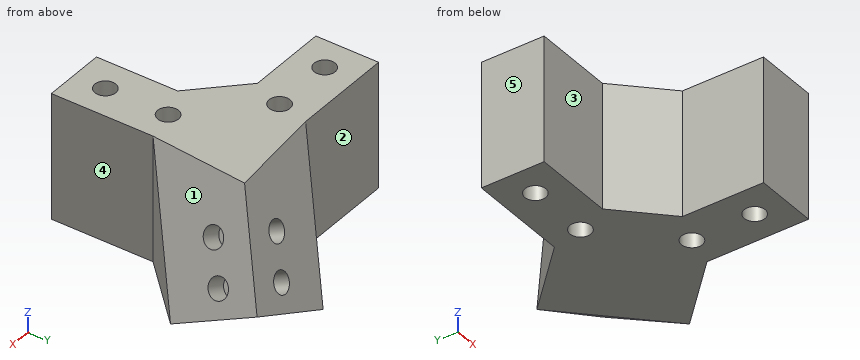
Autodesk Inventor part; units mm, degrees
ref_plane "YZ Plane" through (0, 0, 0) normal (1, 0, 0) x (0, 1, 0)
ref_plane "XZ Plane" through (0, 0, 0) normal (0, 1, 0) x (-1, 0, 0)
ref_plane "XY Plane" through (0, 0, 0) normal (0, 0, 1) x (1, 0, 0)
sketch "スケッチ1" plane through (0, 0, 0) normal (0, 0, 1) x (1, 0, 0)
  line L0 (0, 0) -> (60, 0)
  line L1 (60, 0) -> (60, 60)
  line L2 (60, 60) -> (0, 60)
  line L3 (0, 60) -> (0, 0)
  dimension "d0" = 60
  dimension "d1" = 60
extrude "押し出し1" add sketch "スケッチ1" along normal blind 30
sketch "スケッチ2" plane through (0, 0, 30) normal (0, 0, 1) x (1, 0, 0)
  line L0 (60, 0) -> (60, 60)
  line L1 (60, 60) -> (0, 60)
  point P0 (0, 0)
  point P1 (22, 49.5)
  point P2 (37, 49.5)
  point P3 (52.5, 34)
  point P4 (52.5, 19)
  dimension "d4" = 7.5
  dimension "d5" = 7.5
  dimension "d6" = 10.5
  dimension "d7" = 10.5
  dimension "d8" = 15
  dimension "d9" = 15
  dimension "d10" = 23
  dimension "d11" = 26
hole "穴1" at (22, 49.5, 30) at (37, 49.5, 30) at (52.5, 34, 30) at (52.5, 19, 30) direction (0, 0, -1) diameter 5 end through all
sketch "スケッチ3" plane through (0, 0, 30) normal (0, 0, 1) x (1, 0, 0)
  line L0 (22, 49.5) -> (37, 49.5)
  circle A0 centre (52.5, 34) radius 2.5
  line L1 (37, 49.5) -> (52.5, 34)
  line L2 (52.5, 34) -> (52.5, 19)
  line L3 (22, 49.5) -> (22, 19)
  line L4 (22, 19) -> (52.5, 19)
  line L5 (60, 37.1066) -> (40.1066, 57)
  line L6 (40.1066, 57) -> (14.5, 57)
  line L7 (14.5, 57) -> (14.5, 11.5)
  line L8 (14.5, 11.5) -> (60, 11.5)
  line L9 (60, 11.5) -> (60, 37.1066)
  line L10 (14.5, 57) -> (44.5, 57)
  line L11 (44.5, 57) -> (44.5, 42)
  line L12 (44.5, 42) -> (14.5, 42)
  line L13 (14.5, 42) -> (14.5, 57)
  line L14 (60, 11.5) -> (45, 11.5)
  line L15 (45, 11.5) -> (45, 41.5)
  line L16 (45, 41.5) -> (60, 41.5)
  line L17 (60, 41.5) -> (60, 11.5)
  circle A1 centre (52.5, 19) radius 2.5
  circle A2 centre (52.5, 34) radius 2.5
  circle A3 centre (37, 49.5) radius 2.5
  circle A4 centre (22, 49.5) radius 2.5
  line L18 (60, 0) -> (60, 60)
  line L19 (60, 60) -> (0, 60)
  line L20 (0, 60) -> (0, 0)
  line L21 (0, 0) -> (60, 0)
  line L22 (14.5, 42) -> (45, 11.5)
  line L23 (24.0029, 51.8905) -> (54.5029, 21.3905)
  line L24 (38.7868, 57) -> (60, 35.7868)
  point P0 (52.5, 26.5)
  point P1 (45, 19)
  point P2 (22, 42)
  point P3 (39.2529, 36.6405)
  point P4 (45, 30.8934)
  point P5 (33.8934, 42)
  dimension "d19" = 7.5
  dimension "d20" = 7.5
  dimension "d21" = 7.5
  dimension "d22" = 30
  dimension "d23" = 30
  dimension "d50" = 7.5
  dimension "d52" = 30
extrude "押し出し2" cut sketch "スケッチ3" against normal blind 30 contours L12 L23 L15 L4 L22 L3 | L3 L22 L12 | L22 L4 L3 | L3 L4 L22 L8 L7 | L7 L8 L18 L21 L20 L19 L16 L5 L11 L10 L6 | L4 L15 L22 | L24 L6 L5 L11 | L11 L5 L16 L24 | L16 L5 L9 L24 | L5 L10 L11 | L16 L17 L5
sketch "スケッチ15" plane through (60, 35.7868, 0) normal (0.7071068, 0.7071068, 0) x (-0.7071068, 0.7071068, 0)
  line L0 (0, 30) -> (30, 30)
  line L1 (0, 0) -> (0, 30)
  line L2 (30, 0) -> (0, 0)
  line L3 (30, 30) -> (30, 0)
  point P0 (17.1213, 0)
extrude "押し出し11" add sketch "スケッチ15" along normal blind 30
sketch "スケッチ16" plane through (60, 35.7868, 30) normal (0.7071068, -0.7071068, 0) x (-0.7071068, -0.7071068, 0)
  line L0 (0, 30) -> (0, 0)
  line L1 (0, 30) -> (-30, 30)
  line L2 (-30, 0) -> (-30, 30)
  line L3 (0, 0) -> (-30, 0)
  line L4 (0, 0) -> (-30.762, 43.9327)
  point P0 (67.7315, 30)
  point P1 (-21.0062, 30)
  dimension "d97" = 55
extrude "押し出し12" cut sketch "スケッチ16" against normal blind 30 contours L3 L2 L1 L4
sketch "スケッチ25" plane through (60, 35.7868, 30) normal (0.579228, 0.579228, 0.5735764) x (0.7071068, -0.7071068, 0)
  line L0 (0, 36.6232) -> (0, 0)
  line L1 (-30, 36.6232) -> (0, 36.6232)
  line L2 (-30, 0) -> (-30, 36.6232)
  line L3 (0, 0) -> (-30, 0)
  point P0 (-17.1213, -14.2746)
extrude "押し出し17" add sketch "スケッチ25" along normal blind 30
sketch "スケッチ26" plane through (74.8536, 50.6404, 0) normal (0.4055798, 0.4055798, -0.819152) x (-0.579228, -0.579228, -0.5735764)
  line L0 (0, 30) -> (0, 0)
  line L1 (0, 30) -> (-30, 30)
  line L2 (-30, 0) -> (-30, 30)
  line L3 (0, 0) -> (-30, 0)
  line L4 (0, 0) -> (-30, 30)
  line L5 (0, 30) -> (-30, 0)
  point P0 (72.6897, 17.1213)
  point P1 (-15, 15)
extrude "押し出し18" cut sketch "スケッチ26" against normal through all contours L5 L4 L1 | L3 L5 L4 | L4 L5 L2
sketch "スケッチ27" plane through (74.8536, 50.6404, 0) normal (0.909576, -0.090424, 0.4055798) x (0.4055798, 0.4055798, -0.819152)
  point P0 (-50.8979, -39.2928)
sketch "スケッチ28" plane through (0, 0, 30) normal (0, 0, 1) x (1, 0, 0)
  line L0 (3.3303, 1.5204) -> (87.3121, 1.5204)
  line L1 (87.3121, 1.5204) -> (87.3121, 89.4116)
  line L2 (87.3121, 89.4116) -> (3.3303, 89.4116)
  line L3 (3.3303, 89.4116) -> (3.3303, 1.5204)
  point P0 (0, 0)
extrude "押し出し19" cut sketch "スケッチ28" along normal blind 100
sketch "スケッチ29" plane through (74.8536, 50.6404, 0) normal (0.909576, -0.090424, 0.4055798) x (0.4055798, 0.4055798, -0.819152)
  line L0 (-36.6232, 21.2132) -> (-26.1201, 21.2132)
  line L1 (0, 21.2132) -> (0, 0)
  line L2 (-26.1201, 21.2132) -> (0, 21.2132)
  line L3 (0, 21.2132) -> (0, 0)
  line L4 (0, 0) -> (-26.1201, 0)
  line L5 (-26.1201, 0) -> (-26.1201, 21.2132)
  point P0 (-50.8979, -39.2928)
  point P1 (-16.1201, 12.4132)
  point P2 (-6.1201, 12.4132)
  dimension "d104" = 10
  dimension "d105" = 10
  dimension "d106" = 8.8
  dimension "d107" = 8.8
hole "穴4" at (67.1932, 55.3932, 18.2394) at (71.249, 59.449, 10.0479) direction (-0.909576, 0.090424, -0.4055798) diameter 5 depth 5
sketch "スケッチ30" plane through (53.6404, 71.8536, 0) normal (-0.090424, 0.909576, 0.4055798) x (0.909576, -0.090424, 0.4055798)
  line L0 (21.2132, 0) -> (21.2132, -26.1201)
  line L1 (-12.1674, -12.0487) -> (0, 0)
  line L2 (21.2132, -26.1201) -> (0, -26.1201)
  line L3 (0, -26.1201) -> (0, 0)
  line L4 (0, 0) -> (21.2132, 0)
  line L5 (21.2132, 0) -> (21.2132, -26.1201)
  point P0 (-42.2928, -50.8979)
  point P1 (12.4132, -16.1201)
  point P2 (12.4132, -6.1201)
  dimension "d115" = 10
  dimension "d116" = 10
  dimension "d117" = 8.8
  dimension "d118" = 8.8
hole "穴5" at (58.3932, 64.1932, 18.2394) at (62.449, 68.249, 10.0479) direction (0.090424, -0.909576, -0.4055798) diameter 5 depth 5
equation "\"d20\" = d19"
equation "\"d23\" = d22"
properties part number "EX-L-Connect-50deg"
Geometry check sheet. Reference: the model listing, model coordinates, mm. Face numbers are marked on the shaded views. A direction names the side the tool comes from. Round coordinates to 2 decimals unless told otherwise and drop trailing zeros. Loops run counter-clockwise (first coordinate to the right, second up) from the corner with the lowest first, then second, coordinate; pieces in that order, holes last. Notation, with made-up numbers: (59.25, 1.5) - (94.25, 1.5) arc R26 cw to (94.25, 27.5) - close; hole circle Ø3 at (54, 43). An arc over 180 degrees is marked (long way). Write each question's results on one line, items separated by ' | '. Start each with the question number.
Q1. Cross-section at C-C on z = 4.5. Enter the section's corners in (x, y), and give its area (3 significant figures).
Q2. Gauge pin test, flat ends, axial feed: P1, Ø7.5, axis at x = 26, z = 15.5, coming from the +Y side; P2, Ø3, axis at x = 22, y = 49.5, coming from the -Z side; P3, Ø4, axis at x = 68, z = 8.5, coming from the -Y side; P4, Ø9.5, axis at y = 21.5, z = 17, coming from the -X side. Record the tip position at first contact, or that the pin passes through.
Q3. Cross-section at B-B on y = 34. Enter the section's corners in (x, z).
Q4. Access from +Z, -Z, +X, -X, +Y, -Y to the whole of each face (thin tool, end or side, straight path). Record for the marked faces 1, 2, 3, 4 and 5.
Q5. Cross-section at D-D on x = 52.5. Enter the section's corners in (y, z).
Q6. Cross-section at A-A on x = 22. Enter the section's corners in (y, z).
Q7. Thickness scan on line 1 (Y direction, x = 52.5, z = 15.75); line 2 (Y direction, x = 52.5, z = 15.5); line 3 (X direction, y = 51.5, z = 19). Record the ranges inside material, lowest first. Write a range as [from, to].
Answers below:
1) outline: (14.5, 42) - (33.89, 42) - (45, 30.89) - (45, 11.5) - (60, 11.5) - (60, 35.79) - (72.63, 48.41) - (73.85, 60.73) - (63.73, 70.85) - (51.41, 69.63) - (38.79, 57) - (14.5, 57) - close; hole circle Ø5 at (22, 49.5); hole circle Ø5 at (37, 49.5); hole circle Ø5 at (52.5, 19); hole circle Ø5 at (52.5, 34) | area: 1,650 mm²
2) P1: stops at y = 57 | P2: passes through | P3: stops at y = 41.79 | P4: stops at x = 45
3) outline: (41.89, 0) - (50, 0) - (50, 30) - (41.89, 30) - close; (55, 0) - (60, 0) - (60, 30) - (55, 30) - close
4) face 1: +Z, +X, -Y | face 2: +Z, -Z, -X, +Y | face 3: +Z, -Z, -X, -Y | face 4: +Z, -Z, +X, -Y | face 5: +Z, -Z, -X, +Y, -Y
5) outline: (11.5, 0) - (16.5, 0) - (16.5, 30) - (11.5, 30) - close; (21.5, 0) - (31.5, 0) - (31.5, 30) - (21.5, 30) - close; (36.5, 0) - (70.71, 0) - (70.71, 2.3) - (58.36, 30) - (36.5, 30) - close
6) outline: (42, 0) - (47, 0) - (47, 30) - (42, 30) - close; (52, 0) - (57, 0) - (57, 30) - (52, 30) - close
7) line 1: y = [11.5, 16.5], [21.5, 31.5], [36.5, 64.72] | line 2: y = [11.5, 16.5], [21.5, 31.5], [36.5, 64.83] | line 3: x = [14.5, 20.5], [23.5, 35.5], [38.5, 66.47]
